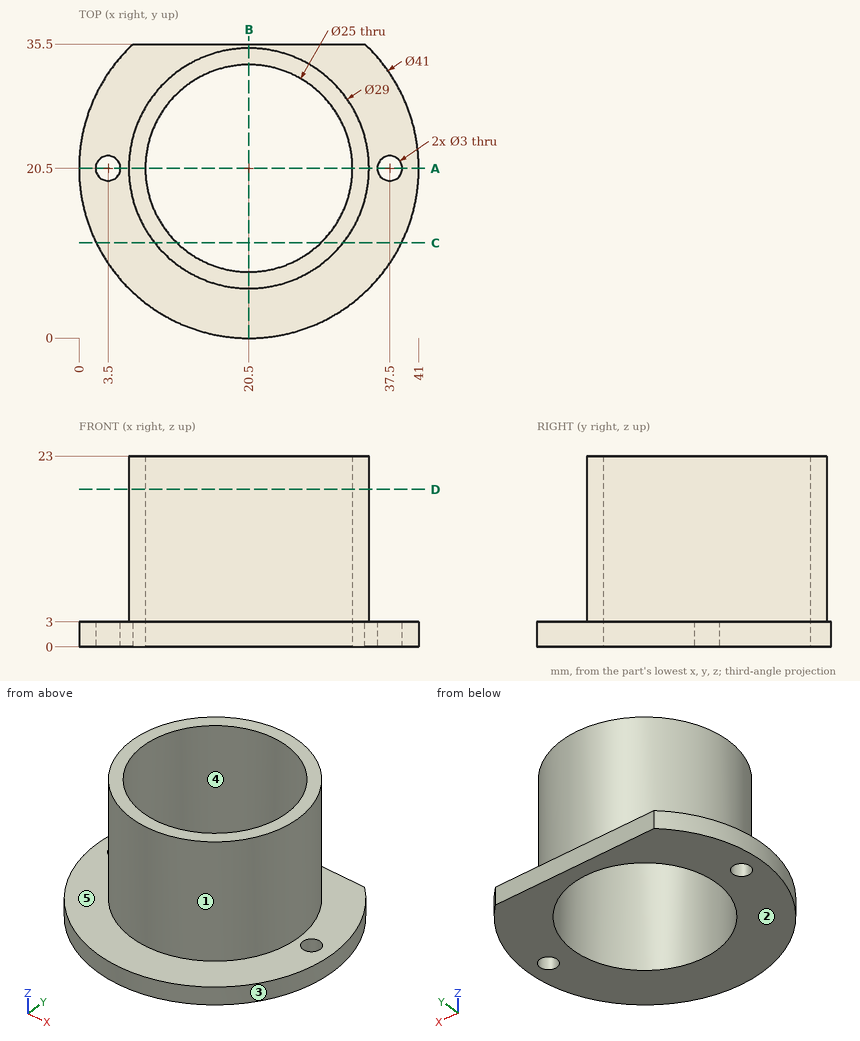
Check sheet for the drawn part. Datum: minimum x, y, z corner. Units: mm. A direction names the side the tool comes from. Round coordinates to 2 decimals unless told otherwise and drop trailing zeros. Order: outer loops, then holes, each group sorted by start corner. A loop starts at its lowest first (then second) coordinate and runs counter-clockwise, first axis right, second up. Notation, with made-up numbers: (-4, 0.25) -> (3, 0.25) arc R33 ccw to (3, 32.25) -> close; hole circle Ø8 at (78, -25.75). An arc over 180 degrees is marked (long way). Put each result on its own line as item: value. Start each with the question number.
(1) Tool access check on the marked faces 1 and 2. Record the directions out of +Z, -Z, +X, -X, +Y, -Y that give a thin tool (end or side, any length) a straight path to the whole face; none if there is none.
(2) Section check C-C (y = 11.5). Enter the section's corners in (x, z).
(3) Material ranges on line 1 along Y through (x, z) = (20, 4.5); line 2 along X through (y, z) = (23, 15.5); line 3 along Y through (x, z) = (37.5, 2.35), recorded low to high.
(4) Depth check by flat-ended pin: pin 1 Ø1.5 at (x, z) = (31.5, 15) entering from -Y; pin 2 Ø4 at (y, z) = (11.5, 12) entering from -X; pin 3 Ø12 at (y, z) = (17, 8.5) entering from -X. Enter the tip coordinate at first touch or a pass-through.
(5) Section check B-B (x = 20.5). Enter the section's corners in (y, z), then the cut area to 4 significant figures.
(6) Section check D-D (z = 19). Enter the section's corners in (x, y).
(7) Draft check along Y on the marked faces 3, 4 and 5. Enter one of: +Y half, -Y half, draft (parallel to the pull), parting line (faces both ways), or undercut.
(8) Section check A-A (y = 20.5). Enter the section's corners in (x, z).
Completed:
1. face 1: +Z
1. face 2: -Z, +X, -X, +Y, -Y
2. outline: (2.08, 0) -> (11.83, 0) -> (11.83, 23) -> (9.13, 23) -> (9.13, 3) -> (2.08, 3) -> close; (29.17, 0) -> (38.92, 0) -> (38.92, 3) -> (31.87, 3) -> (31.87, 23) -> (29.17, 23) -> close
3. line 1: y = 6.01 to 8.01, 32.99 to 34.99
3. line 2: x = 6.22 to 8.25, 32.75 to 34.78
3. line 3: y = 9.04 to 19, 22 to 31.96
4. pin 1: stops at y = 10.24
4. pin 2: stops at x = 7.8
4. pin 3: stops at x = 0.03
5. outline: (0, 0) -> (8, 0) -> (8, 23) -> (6, 23) -> (6, 3) -> (0, 3) -> close; (33, 0) -> (35.5, 0) -> (35.5, 3) -> (35, 3) -> (35, 23) -> (33, 23) -> close
5. area: 111.5 mm2
6. outline: circle Ø29 at (20.5, 20.5); hole circle Ø25 at (20.5, 20.5)
7. face 3: parting line
7. face 4: undercut
7. face 5: draft
8. outline: (0, 0) -> (2, 0) -> (2, 3) -> (0, 3) -> close; (5, 0) -> (8, 0) -> (8, 23) -> (6, 23) -> (6, 3) -> (5, 3) -> close; (33, 0) -> (36, 0) -> (36, 3) -> (35, 3) -> (35, 23) -> (33, 23) -> close; (39, 0) -> (41, 0) -> (41, 3) -> (39, 3) -> close
